from build123d import *

# Parameters (mm, degrees)
F1_DEPTH = 38.1
F2_R     = 6.35


with BuildPart() as f1:
    # F0 (on Top) → F1 (new body)
    with BuildSketch(Plane.XY):
        Polygon((-31.75, 47.625), (0, 47.625), (0, 60.325), (-38.1, 60.325), (-47.625, 47.625), align=None)
        Polygon((0, 47.625), (31.75, 47.625), (47.625, 47.625), (38.1, 60.325), (0, 60.325), align=None)
        with BuildLine():
            ThreePointArc((-57.15, 34.925), (-45.9490316571, 44.2730633142), (-31.75, 47.625))
            Line((-31.75, 47.625), (-47.625, 47.625))
            Line((-47.625, 47.625), (-57.15, 34.925))
        make_face()
        with BuildLine():
            Line((0, 34.925), (0, 47.625))
            Line((0, 47.625), (-31.75, 47.625))
            ThreePointArc((-31.75, 47.625), (-45.9490316571, 44.2730633142), (-57.15, 34.925))
            Line((-57.15, 34.925), (0, 34.925))
        make_face()
        with BuildLine():
            ThreePointArc((57.15, 34.925), (45.9490316571, 44.2730633142), (31.75, 47.625))
            Line((31.75, 47.625), (0, 47.625))
            Line((0, 47.625), (0, 34.925))
            Line((0, 34.925), (57.15, 34.925))
        make_face()
        with BuildLine():
            Line((47.625, 47.625), (31.75, 47.625))
            ThreePointArc((31.75, 47.625), (45.9490316571, 44.2730633142), (57.15, 34.925))
            Line((57.15, 34.925), (47.625, 47.625))
        make_face()
        with BuildLine():
            ThreePointArc((58.801, 32.4974516543), (58.0035730519, 33.7303185916), (57.15, 34.925))
            Line((57.15, 34.925), (0, 34.925))
            Line((0, 34.925), (-57.15, 34.925))
            ThreePointArc((-57.15, 34.925), (-58.0035730519, 33.7303185916), (-58.801, 32.4974516543))
            Line((-58.801, 32.4974516543), (-58.801, -0.7474516543))
            ThreePointArc((-58.801, -0.7474516543), (-55.2145879783, -5.513679506), (-50.8, -9.525))
            Line((-50.8, -9.525), (-50.8, -47.625))
            Line((-50.8, -47.625), (0, -47.625))
            Line((0, -47.625), (50.8, -47.625))
            Line((50.8, -47.625), (50.8, -9.525))
            ThreePointArc((50.8, -9.525), (55.2145879783, -5.513679506), (58.801, -0.7474516543))
            Line((58.801, -0.7474516543), (58.801, 32.4974516543))
        make_face()
        with BuildLine():
            ThreePointArc((58.801, -0.7474516543), (63.5, 15.875), (58.801, 32.4974516543))
            Line((58.801, 32.4974516543), (58.801, -0.7474516543))
        make_face()
        with BuildLine():
            Line((-58.801, -0.7474516543), (-58.801, 32.4974516543))
            ThreePointArc((-58.801, 32.4974516543), (-63.5, 15.875), (-58.801, -0.7474516543))
        make_face()
    extrude(amount=F1_DEPTH)

    # F2
    f2_edges = [f1.edges().sort_by_distance(p)[0] for p in [
        (-50.8, -47.625, 19.05),
        (50.8, -47.625, 19.05),
        (50.8, -9.525, 19.05),
        (-50.8, -9.525, 19.05),
        (-38.1, 60.325, 19.05),
        (38.1, 60.325, 19.05),
    ]]
    fillet(f2_edges, radius=F2_R)


solid = f1.part
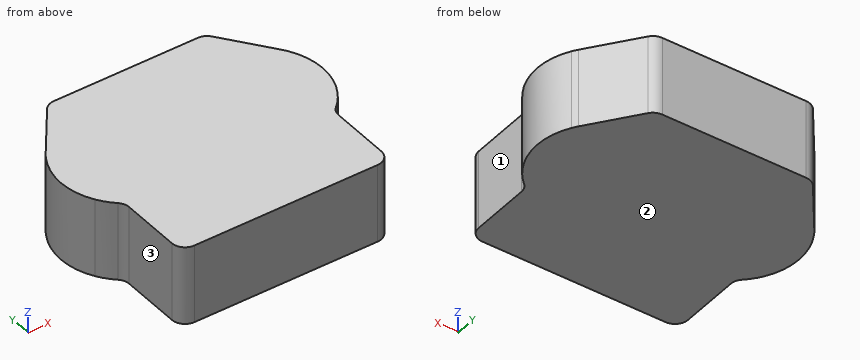
For this review, take the finished solid that the model builds, in its own axes (mm). Face numbers are marked on the shaded views. A direction names the side the tool comes from. Coordinates: 2 decimals unless noted, no trailing zeros. Loops run counter-clockwise (first coordinate to the right, second up) from the corner with the lowest first, then second, coordinate; pieces in that order, holes last. Notation, with made-up numbers: (-34.75, 89) - (-3.75, 89) arc R30 ccw to (-3.75, 127) - close; hole circle Ø7 at (40, -14). An arc over 180 degrees is marked (long way). Return JSON: item names as keys, results as strings.
Item 1: Insertion check: pin 1 (2 mm diameter, centred on y = 19.5, z = 14.5, fed in from -X); pin 2 (4 mm diameter, centred on y = -19, z = 21.5, fed in from +X). Each pin has a flat end and moves straight along its axis. Give the tip position at first contact, or say it passes through.
Determined:
{"pin 1": "stops at x = -63.39", "pin 2": "stops at x = 50.8"}
Item 2: For the marked faces 1, 2 and 3, list the 3-axis set-ups (+Z, -Z, +X, -X, +Y, -Y) from which the entire face can be reached by the end or side of a thin tool; tool diameter is ignored.
Determined:
{"face 1": "+Z, -Z, +X, -Y", "face 2": "-Z, +X, -X, +Y, -Y", "face 3": "+Z, -Z, -X, -Y"}
Item 3: Take a section at C-C (x = -43). Give the boundary of the cut face in (y, z) (3 decimals), then the cut area to 3 significant figures.
Determined:
{"outline": "(-47.625, 0) - (53.792, 0) - (53.792, 38.1) - (-47.625, 38.1) - close", "area": "3,860 mm2"}
Item 4: Take a section at B-B (y = -29.5). Give the boundary of the cut face in (x, z).
Determined:
{"outline": "(-50.8, 0) - (50.8, 0) - (50.8, 38.1) - (-50.8, 38.1) - close"}
Item 5: For line 1 (X direction, y = -19, z = 33.5); line 2 (X direction, y = 54, z = 19.5); line 3 (Y direction, x = 56.5, z = 33.5), list the stretches that pass through material, from the lowest coordinate up.
Determined:
{"line 1": "x = -50.8 to 50.8", "line 2": "x = -42.84 to 42.84", "line 3": "y = -4.01 to 35.79"}
Item 6: Take a section at A-A (z = 15.5). Give the boundary of the cut face in (x, y) (3 decimals), then the cut area to 3 significant figures.
Determined:
{"outline": "(-57.15, 34.925) arc R31.75 ccw to (-52.917, -7.79) arc R6.35 cw to (-50.8, -12.523) - (-50.8, -41.275) arc R6.35 ccw to (-44.45, -47.625) - (44.45, -47.625) arc R6.35 ccw to (50.8, -41.275) - (50.8, -12.523) arc R6.35 cw to (52.917, -7.79) arc R31.75 ccw to (57.15, 34.925) - (40.005, 57.785) arc R6.35 ccw to (34.925, 60.325) - (-34.925, 60.325) arc R6.35 ccw to (-40.005, 57.785) - close", "area": "11,600 mm2"}
